Study the drawing (mm; zero at the part's minimum x, y, z) and answer. Coordinates: 2 decimals unless noted, no trailing zeros. Order: outer loops, then holes, each group sorted by start corner. A loop starts at its lowest first (then second) coordinate and runs counter-clockwise, first axis right, second up. Notation, with made-up numbers: M 84,25.5 L 124,25.5 A17 cw 124,54.5 Z; hole C 61.25,62.25 d8. An arc over 180 degrees is marked long. Put each result on its own line as item: value.
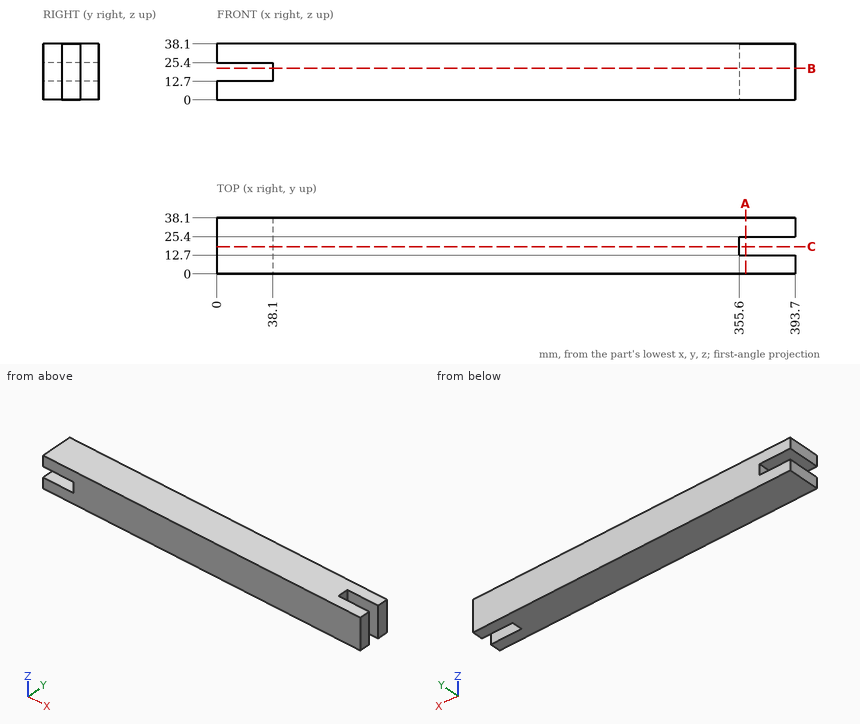
Q1. Find section B-B on z = 21.5. Write down the section's boundary in (x, y), plus the area to 3 significant figures.
Answers below:
outline: M 38.1,0 L 393.7,0 L 393.7,12.7 L 355.6,12.7 L 355.6,25.4 L 393.7,25.4 L 393.7,38.1 L 38.1,38.1 Z
area: 13,100 mm^2
Q2. Find section A-A on x = 360. Write down the section's boundary in (y, z).
Answers below:
outline: M 0,0 L 12.7,0 L 12.7,38.1 L 0,38.1 Z; M 25.4,0 L 38.1,0 L 38.1,38.1 L 25.4,38.1 Z
Q3. Given pin 1 (19 mm diameter, centred on x = 382, z = 15, fed in from -Y); pin 2 (6.5 mm diameter, centred on y = 22.5, z = 21, fed in from -X); pin 3 (6 mm diameter, centred on y = 17.5, z = 21.5, fed in from +X), each flat-ended and moving along its own axis, determine where each tip first touches the part or whether it passes through.
Answers below:
pin 1: stops at y = 0
pin 2: stops at x = 38.1
pin 3: stops at x = 355.6
Q4. Consider line 1 along Z through (x, y) = (23.5, 22); line 2 along X through (y, z) = (19, 25). Determine where each line is inside the solid, lowest interval first.
Answers below:
line 1: z = 0 to 12.7, 25.4 to 38.1
line 2: x = 38.1 to 355.6
Q5. Find section C-C on y = 18.5. Write down the section's boundary in (x, z), plus the area to 3 significant figures.
Answers below:
outline: M 0,0 L 355.6,0 L 355.6,38.1 L 0,38.1 L 0,25.4 L 38.1,25.4 L 38.1,12.7 L 0,12.7 Z
area: 13,100 mm^2
